Could you check a few things on this model? Use its own coordinates, in mm. A direction names the side the tool comes from. Round coordinates to 2 decimals unless told otherwise and drop trailing zeros. Loops run counter-clockwise (first coordinate to the right, second up) from the corner with the lowest first, then second, coordinate; pieces in that order, holes last. Notation, with made-up numbers: (33.25, 20) -> (61.25, 20) arc R24 cw to (61.25, 48) -> close; hole circle Ø10 at (88, 72.25). An arc over 180 degrees is marked (long way). Write each question's results on one line, items separated by ' | '.
from build123d import *

# Parameters (mm, degrees)
REVOLUCI_N1_OUTLINE_R     = 32.5
REVOLUCI_N1_DEPTH         = 8.5
REVOLUCI_N1_START         = 8.5
REVOLUCI_N1_2_OUTLINE_R   = 32.5
REVOLUCI_N1_2_OUTLINE_R_2 = 22.5
REVOLUCI_N1_2_OUTLINE_R_3 = 9.5
REVOLUCI_N1_2_DEPTH       = 2.5
CROQUIS2_R                = 7
CROQUIS2_R_2              = 1.5
CORTAR_EXTRUIR1_DEPTH     = 16
CORTAR_EXTRUIR2_START     = -16
CORTAR_EXTRUIR2_DEPTH     = 16
CORTAR_EXTRUIR4_DEPTH     = 2.5
CROQUIS7_R                = 3.25
CORTAR_EXTRUIR6_DEPTH     = 2.5
CROQUIS9_R                = 24.21
CROQUIS9_R_2              = 18.21
CORTAR_EXTRUIR7_DEPTH     = 2.5


# Read off the part's stored shape, not the designer's step: Revolución1
with BuildPart() as part:
    # Revolución1 outline → Revolución1 (new body)
    with BuildSketch(Plane.YZ):
        Circle(REVOLUCI_N1_OUTLINE_R)
    extrude(amount=REVOLUCI_N1_DEPTH)

    # Revoluci_n1 2 outline → Revoluci_n1 2 (add)
    # profile 1 of 2: a face of its own
    with BuildSketch(Plane.YZ.offset(REVOLUCI_N1_START)):
        Circle(REVOLUCI_N1_2_OUTLINE_R)
        Circle(REVOLUCI_N1_2_OUTLINE_R_2, mode=Mode.SUBTRACT)
    # profile 2 of 2: a face of its own
    with BuildSketch(Plane.YZ.offset(REVOLUCI_N1_START)):
        Circle(REVOLUCI_N1_2_OUTLINE_R_3)
    extrude(amount=REVOLUCI_N1_2_DEPTH)

    # Croquis2 → Cortar-Extruir1 (cut)
    with BuildSketch(Plane(origin=(11, 0, 0), x_dir=(0, 0, -1), z_dir=(1, 0, 0))):
        Circle(CROQUIS2_R)
        with Locations((25.406687144, -10.52379439)):
            Circle(CROQUIS2_R_2)
        with Locations((10.52379439, -25.406687144)):
            Circle(CROQUIS2_R_2)
        with Locations((-10.52379439, -25.406687144)):
            Circle(CROQUIS2_R_2)
        with Locations((-25.406687144, -10.52379439)):
            Circle(CROQUIS2_R_2)
        with Locations((-25.406687144, 10.52379439)):
            Circle(CROQUIS2_R_2)
        with Locations((25.406687144, 10.52379439)):
            Circle(CROQUIS2_R_2)
    extrude(amount=-CORTAR_EXTRUIR1_DEPTH, mode=Mode.SUBTRACT)

    # Croquis3 → Cortar-Extruir2 (cut)
    with BuildSketch(Plane(origin=(11, 0, 0), x_dir=(0, 0, -1), z_dir=(1, 0, 0)).offset(CORTAR_EXTRUIR2_START)):
        with BuildLine():
            Line((-22.980970389, 22.980970389), (-15.909902577, 15.909902577))
            ThreePointArc((-15.909902577, 15.909902577), (0, 22.5), (15.909902577, 15.909902577))
            Line((15.909902577, 15.909902577), (22.980970389, 22.980970389))
            ThreePointArc((22.980970389, 22.980970389), (0, 32.5), (-22.980970389, 22.980970389))
        make_face()
    extrude(amount=CORTAR_EXTRUIR2_DEPTH, mode=Mode.SUBTRACT)

    # Croquis5 → Cortar-Extruir4 (cut)
    with BuildSketch(Plane(origin=(11, 0, 0), x_dir=(0, 0, -1), z_dir=(1, 0, 0))):
        with BuildLine():
            ThreePointArc((31.7, 0), (27.5, 4.2), (23.3, 0))
            Line((23.3, 0), (31.7, 0))
        make_face()
        with BuildLine():
            Line((31.7, 0), (23.3, 0))
            ThreePointArc((23.3, 0), (27.5, -4.2), (31.7, 0))
        make_face()
        with BuildLine():
            ThreePointArc((-31.7, 0), (-27.5, -4.2), (-23.3, 0))
            Line((-23.3, 0), (-31.7, 0))
        make_face()
        with BuildLine():
            Line((-31.7, 0), (-23.3, 0))
            ThreePointArc((-23.3, 0), (-27.5, 4.2), (-31.7, 0))
        make_face()
    extrude(amount=-CORTAR_EXTRUIR4_DEPTH, mode=Mode.SUBTRACT)

    # Croquis7 → Cortar-Extruir6 (cut)
    with BuildSketch(Plane(origin=(11, 0, 0), x_dir=(0, 0, -1), z_dir=(1, 0, 0))):
        with Locations((25.406687144, -10.52379439)):
            Circle(CROQUIS7_R)
        with Locations((10.52379439, -25.406687144)):
            Circle(CROQUIS7_R)
        with Locations((-10.52379439, -25.406687144)):
            Circle(CROQUIS7_R)
        with Locations((-25.406687144, -10.52379439)):
            Circle(CROQUIS7_R)
        with Locations((-25.406687144, 10.52379439)):
            Circle(CROQUIS7_R)
        with Locations((25.406687144, 10.52379439)):
            Circle(CROQUIS7_R)
    extrude(amount=-CORTAR_EXTRUIR6_DEPTH, mode=Mode.SUBTRACT)

    # Croquis9 → Cortar-Extruir7 (cut)
    with BuildSketch(Plane.ZY):
        Circle(CROQUIS9_R)
        Circle(CROQUIS9_R_2, mode=Mode.SUBTRACT)
    extrude(amount=-CORTAR_EXTRUIR7_DEPTH, mode=Mode.SUBTRACT)


solid = part.part
1) I want a section at C-C, the plane x = 10. Give the number of separate pieces and of enclosed holes in the cut face, plus the area to 3 significant figures.
Model answer:
separate pieces: 2 | enclosed holes: 9 | area: 1,120 mm2
2) For faces 4 (the cylindrical face through (4.31, -11.99, 25.73)), 5 (the flat face through (2.5, -18, -4)), 6 (the flat face through (8.5, 10, -27)), 7 (the flat face through (5, 19, -19)), which set-ups out of +Z, -Z, +X, -X, +Y, -Y let a thin tool reach every point of the face, with its end or its side?
Model answer:
face 4: +X, -X | face 5: -X | face 6: +X | face 7: +X, -X, +Y
3) I need wall thicknesses on line 1 (Y direction, x = 7.5, z = 26); line 2 (Y direction, x = 6.5, z = 0); line 3 (Z direction, x = 6.25, y = 11.5). Which ranges of each line are inside material? Lowest first, please.
Model answer:
line 1: y = -19.5 to -11.9, -9.15 to 9.15, 11.9 to 19.5 | line 2: y = -32.5 to -7, 7 to 22.5 | line 3: z = -30.4 to -26.55, -24.27 to 24.27, 26.55 to 30.4
4) I'm going to push flat-ended pins straight in: pin 1 (3.5 mm diameter, centred on y = -25.41, z = 10.52, fed in from +X); pin 2 (6 mm diameter, centred on x = 10, z = 12.5, fed in from +Y); pin 3 (5 mm diameter, centred on y = -25.5, z = -11.5, fed in from +X); pin 4 (6 mm diameter, centred on x = 4.5, z = 14, fed in from -Y). Where does each tip first touch, or does it pass through?
Model answer:
pin 1: stops at x = 8.5 | pin 2: stops at y = 20.2 | pin 3: stops at x = 11 | pin 4: stops at y = -30.58
5) If we mould it in two halves opening along Y, with no side actions, what happens to faces 1 (the cylindrical face through (9.768, 10.667, 28.654)), 2 (the flat face through (11, -4, -6)), 3 (the flat face through (5, 19, 19))? For each: released by +Y, released by -Y, zero draft, split by the parting line, or undercut.
Model answer:
face 1: undercut | face 2: zero draft | face 3: released by +Y
6) I want a section at A-A, the plane z = 0. Write out the boundary of the cut face in (x, y).
Model answer:
outline: (0, -32.5) -> (11, -32.5) -> (11, -22.5) -> (8.5, -22.5) -> (8.5, -9.5) -> (11, -9.5) -> (11, -7) -> (0, -7) -> (0, -18.21) -> (2.5, -18.21) -> (2.5, -24.21) -> (0, -24.21) -> close; (0, 7) -> (11, 7) -> (11, 9.5) -> (8.5, 9.5) -> (8.5, 22.5) -> (2.5, 22.5) -> (2.5, 18.21) -> (0, 18.21) -> close
7) I want a section at D-D, the plane x = 3.5. Write out the boundary of the cut face in (y, z).
Model answer:
outline: (15.91, -15.91) arc R22.5 ccw to (15.91, 15.91) -> (22.98, 22.98) arc R32.5 ccw (long way) to (22.98, -22.98) -> close; hole circle Ø3 at (-25.41, -10.52); hole circle Ø3 at (-25.41, 10.52); hole circle Ø3 at (-10.52, -25.41); hole circle Ø3 at (-10.52, 25.41); hole circle Ø14 at (0, 0); hole circle Ø3 at (10.52, -25.41); hole circle Ø3 at (10.52, 25.41)
